Model file for the job. Use its own axes, mm. Face numbers are marked on the shaded views. Coordinates: 2 decimals unless noted, no trailing zeros. Order: outer loops, then holes, each group sorted by start corner. A loop starts at its lowest first (then second) coordinate and runs counter-clockwise, first axis right, second up. Notation, with made-up numbers: (16.5, 76.25) -> (53.5, 76.25) arc R22 ccw to (53.5, 96.25) -> close; hole circle Ø6 at (56.5, 85.25). An arc over 180 degrees is marked (long way). Write item = value, one per line. Start each with the question number.
Q1. Mould opens along X. For the marked faces 1, 2, 3 and 4 say: +X half, -X half, draft (parallel to the pull), parting line (faces both ways), or undercut.
Q2. Cut at A-A, the plane y = -2.25. List the corners of the cut face in (x, z), plus the area to 3 significant figures.
Q3. Cut at C-C, the plane x = -190.5. List the corners of the cut face in (y, z), plus the area to 4 significant figures.
Q4. Wall check: line 1 (X direction, y = 0.25, z = 3.25); line 2 (Z direction, x = -187, y = -2.5); line 3 (X direction, y = 0, z = 3.25). Give the ranges that are in metal, low to high. Write a range as from..to.
Q5. Flat gauge pin, fed straight in: pin 1 (1.5 mm diameter, centred on x = -181, z = 4.5, fed in from +Y). Where does the tip first touch, or does it go through?
Q6. Cut at D-D, the plane z = 4.5. Give the number of separate pieces and of enclosed holes in the cut face, plus the area to 3 significant figures.
Q7. Cut at B-B, the plane y = 8.25. List the corners of the cut face in (x, z).
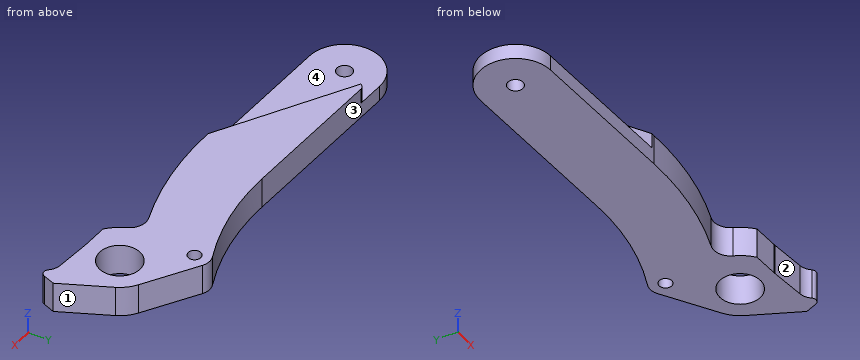
Autodesk Inventor part; units mm, degrees
ref_plane "YZ Plane" through (0, 0, 0) normal (1, 0, 0) x (0, 1, 0)
ref_plane "XZ Plane" through (0, 0, 0) normal (0, 1, 0) x (-1, 0, 0)
ref_plane "XY Plane" through (0, 0, 0) normal (0, 0, 1) x (1, 0, 0)
sketch "スケッチ1" plane through (0, 0, 0) normal (0, 0, 1) x (1, 0, 0)
  circle A0 centre (-145.5257, 0.5882) radius 1.5
  circle A1 centre (-139.5445, -10.0968) radius 1.5
  circle A2 centre (-105.5257, -16.4118) radius 30.1 construction
  line L0 (-170.915, -81.4118) -> (490.0044, -81.4118)
  circle A3 centre (-145.5257, 0.5882) radius 4.025
  circle A4 centre (-139.5445, -10.0968) radius 3
  circle A5 centre (-145.5257, 0.5882) radius 7.025
  line L1 (-146.2365, -6.4007) -> (-139.241, -7.1122)
  line L2 (-139.2044, 3.6529) -> (-134.6999, -5.6381)
  line L3 (-134.6999, -5.6381) -> (-136.7303, -11.1361)
  circle A6 centre (-105.5257, -16.4118) radius 31.1 construction
  line L4 (-145.1707, 7.6042) -> (-210.0877, 10.8882)
  line L5 (-145.8806, -6.4278) -> (-210.7976, -3.1438)
  circle A7 centre (-210.4427, 3.8722) radius 1.5
  circle A8 centre (-210.4427, 3.8722) radius 4.025
  circle A9 centre (-210.4427, 3.8722) radius 7.025
  circle A10 centre (-210.4427, 3.8722) radius 7.525
  line L6 (-206.5907, 10.3366) -> (-181.4786, -4.627)
  circle A11 centre (-199.4194, 13.3524) radius 1.25
  arc A12 (-199.5709, 10.3562) -> (-202.1936, 14.494) centre (-199.4194, 13.3524) ccw
  line L7 (-202.1936, 14.494) -> (-247.2482, 16.7732)
  arc A13 (-289.8377, 39.1951) -> (-247.2482, 16.7732) centre (-244.3571, 73.9244) ccw
  arc A14 (-289.8377, 39.1951) -> (-291.5649, 38.2266) centre (-290.6325, 38.5882) ccw
  arc A15 (-291.5649, 38.2266) -> (-251.8636, 4.9117) centre (-241.4172, 57.674) ccw
  line L8 (-251.8636, 4.9117) -> (-211.807, -3.019)
  line L9 (-209.3045, 11.3106) -> (-204.7936, 10.6204)
  arc A16 (-204.7936, 10.6204) -> (-205.5417, 8.9052) centre (-204.8441, 9.6217) ccw
  line L10 (-210.5022, 11.397) -> (-238.3358, 2.2334)
  point P0 (0, 0)
  point P1 (0, 0)
  point P2 (-146.0589, -6.4188)
  point P3 (-205.8121, 9.8726)
  dimension "d0" = 6
  dimension "d1" = 8.05
  dimension "d2" = 3
  dimension "d3" = 1
  dimension "d4" = 3
  dimension "d5" = 8.05
  dimension "d6" = 3
  dimension "d7" = 0.5
  dimension "d8" = 2.5
  dimension "d9" = 6
  dimension "d10" = 2
  dimension "d11" = 120
  dimension "d12" = 4
  dimension "d13" = 150
  dimension "d14" = 1
  dimension "d15" = 65
  dimension "d16" = 87.382
extrude "押し出し1" add sketch "スケッチ1" along normal blind 6 contours A4 L1 L5 A5 L2 L3 | L5 L6 A16 L4 A5 L1 | A5
extrude "押し出し2" add sketch "スケッチ1" along normal blind 3 contours L5 A10 A16 L6 | L5 A9 A16 A10 | A16 A10 L6 | L6 A10 L4 A16 | A9 | A10 A16 A9 L4 | A8
fillet "フィレット1" radius 1 1 edges at (-136.7303, -11.1361, 3)
sketch "スケッチ2" plane through (0, 0, 6) normal (0, 0, 1) x (1, 0, 0)
  line L0 (-210.7976, -3.1438) -> (-181.4786, -4.627)
  line L1 (-205.8121, 9.8726) -> (-181.4786, -4.627)
  arc A0 (-204.7936, 10.6204) -> (-205.8121, 9.8726) centre (-204.8441, 9.6217) ccw
  line L2 (-204.7936, 10.6204) -> (-210.0877, 10.8882)
  arc A1 (-210.0877, 10.8882) -> (-210.7976, -3.1438) centre (-210.4427, 3.8722) ccw
  circle A2 centre (-210.4427, 3.8722) radius 1.5
  arc A3 (-137.2374, -8.1793) -> (-135.5302, -7.8865) centre (-136.4683, -7.5401) ccw
  line L3 (-135.5302, -7.8865) -> (-134.6999, -5.6381)
  line L4 (-134.6999, -5.6381) -> (-139.2044, 3.6529)
  arc A4 (-139.2044, 3.6529) -> (-145.1707, 7.6042) centre (-145.5257, 0.5882) ccw
  line L5 (-145.1707, 7.6042) -> (-204.7936, 10.6204)
  arc A5 (-204.7936, 10.6204) -> (-205.8121, 9.8726) centre (-204.8441, 9.6217) ccw
  line L6 (-205.8121, 9.8726) -> (-181.4786, -4.627)
  line L7 (-181.4786, -4.627) -> (-146.0589, -6.4188)
  line L8 (-146.0589, -6.4188) -> (-146.2365, -6.4007)
  arc A6 (-146.2365, -6.4007) -> (-145.8806, -6.4278) centre (-145.5257, 0.5882) ccw
  line L9 (-145.8806, -6.4278) -> (-146.0589, -6.4188)
  line L10 (-146.0589, -6.4188) -> (-139.241, -7.1122)
  arc A7 (-137.2374, -8.1793) -> (-139.241, -7.1122) centre (-139.5445, -10.0968) ccw
  circle A8 centre (-145.5257, 0.5882) radius 4.025
  arc A9 (-204.7936, 10.6204) -> (-205.8121, 9.8726) centre (-204.8441, 9.6217) ccw
  line L11 (-204.6925, 12.6179) -> (-209.9867, 12.8857)
  arc A10 (-209.9867, 12.8857) -> (-210.8986, -5.1413) centre (-210.4427, 3.8722) ccw
  arc A11 (-182.0757, -6.5994) -> (-181.4786, -4.627) centre (-182.022, -5.539) ccw
  line L12 (-210.8986, -5.1413) -> (-182.0757, -6.5994)
  arc A12 (-204.7936, 10.6204) -> (-204.6925, 12.6179) centre (-204.743, 11.6191) ccw
  point P0 (0, 0)
  dimension "d22" = 2
sketch "スケッチ3" plane through (0, 0, 6) normal (0, 0, 1) x (1, 0, 0)
  arc A0 (-137.2374, -8.1793) -> (-135.5302, -7.8865) centre (-136.4683, -7.5401) ccw
  line L0 (-135.5302, -7.8865) -> (-134.6999, -5.6381)
  line L1 (-134.6999, -5.6381) -> (-139.2044, 3.6529)
  arc A1 (-139.2044, 3.6529) -> (-145.1707, 7.6042) centre (-145.5257, 0.5882) ccw
  line L2 (-145.1707, 7.6042) -> (-204.7936, 10.6204)
  arc A2 (-204.7936, 10.6204) -> (-205.8121, 9.8726) centre (-204.8441, 9.6217) ccw
  line L3 (-205.8121, 9.8726) -> (-181.4786, -4.627)
  line L4 (-181.4786, -4.627) -> (-146.0589, -6.4188)
  line L5 (-146.0589, -6.4188) -> (-146.2365, -6.4007)
  arc A3 (-146.2365, -6.4007) -> (-145.8806, -6.4278) centre (-145.5257, 0.5882) ccw
  line L6 (-145.8806, -6.4278) -> (-146.0589, -6.4188)
  line L7 (-146.0589, -6.4188) -> (-139.241, -7.1122)
  arc A4 (-137.2374, -8.1793) -> (-139.241, -7.1122) centre (-139.5445, -10.0968) ccw
  circle A5 centre (-145.5257, 0.5882) radius 4.025
  point P0 (0, 0)
extrude "押し出し3" add sketch "スケッチ3" against normal blind 6 contours L5 A3 L6
sketch "スケッチ4" plane through (0, 0, 6) normal (0, 0, 1) x (1, 0, 0)
  line L0 (-146.0589, -6.4188) -> (-139.241, -7.1122)
  arc A0 (-137.2374, -8.1793) -> (-139.241, -7.1122) centre (-139.5445, -10.0968) ccw
  arc A1 (-137.2374, -8.1793) -> (-135.5302, -7.8865) centre (-136.4683, -7.5401) ccw
  line L1 (-135.5302, -7.8865) -> (-134.6999, -5.6381)
  line L2 (-134.6999, -5.6381) -> (-139.2044, 3.6529)
  arc A2 (-139.2044, 3.6529) -> (-145.1707, 7.6042) centre (-145.5257, 0.5882) ccw
  line L3 (-145.1707, 7.6042) -> (-204.7936, 10.6204)
  arc A3 (-204.7936, 10.6204) -> (-205.8121, 9.8726) centre (-204.8441, 9.6217) ccw
  line L4 (-205.8121, 9.8726) -> (-181.4786, -4.627)
  line L5 (-181.4786, -4.627) -> (-146.0589, -6.4188)
  circle A4 centre (-145.5257, 0.5882) radius 4.025
  arc A5 (-153.4999, -3.002) -> (-157.5446, -1.2714) centre (-156.4634, -4.3363) ccw
  arc A6 (-180.854, -4.6586) -> (-157.5446, -1.2714) centre (-177.7808, 56.0903) ccw
  line L6 (-181.4786, -4.627) -> (-146.0589, -6.4188)
  circle A7 centre (-139.5445, -10.0968) radius 3
  arc A8 (-153.4999, -3.002) -> (-151.0823, -6.1647) centre (-145.5257, 0.5882) ccw
  line L7 (-145.1707, 7.6042) -> (-204.7936, 10.6204)
  arc A9 (-176.1768, 9.1728) -> (-154.4643, 13.0367) centre (-173.6978, 58.1782) ccw
  arc A10 (-151.6818, 12.8103) -> (-154.4643, 13.0367) centre (-153.2884, 10.2768) ccw
  line L8 (-151.6818, 12.8103) -> (-141.7636, 6.5209)
  circle A11 centre (-153.2884, 10.2768) radius 1.25
  circle A12 centre (-139.5445, -10.0968) radius 3.5
  point P0 (0, 0)
  point P1 (-176.1768, 9.1728)
  dimension "d25" = 3.25
  dimension "d26" = 95
  dimension "d27" = 3
  dimension "d28" = 2.5
  dimension "d29" = 0.5
extrude "押し出し4" cut sketch "スケッチ4" against normal blind 6 contours L5 A6 A5 A8
extrude "押し出し5" add sketch "スケッチ4" against normal blind 6 contours A2 L3 A9 A10 L8
sketch "スケッチ5" plane through (0, 0, 6) normal (0, 0, 1) x (1, 0, 0)
  circle A0 centre (-153.2884, 10.2768) radius 1.25
  circle A1 centre (-145.5257, 0.5882) radius 4.025
  arc A2 (-180.854, -4.6586) -> (-157.5446, -1.2714) centre (-177.7808, 56.0903) ccw
  arc A3 (-153.4999, -3.002) -> (-157.5446, -1.2714) centre (-156.4634, -4.3363) ccw
  arc A4 (-153.4999, -3.002) -> (-151.0823, -6.1647) centre (-145.5257, 0.5882) ccw
  line L0 (-151.0823, -6.1647) -> (-146.0589, -6.4188)
  line L1 (-146.0589, -6.4188) -> (-139.241, -7.1122)
  arc A5 (-137.2374, -8.1793) -> (-139.241, -7.1122) centre (-139.5445, -10.0968) ccw
  arc A6 (-137.2374, -8.1793) -> (-135.5302, -7.8865) centre (-136.4683, -7.5401) ccw
  line L2 (-135.5302, -7.8865) -> (-134.6999, -5.6381)
  line L3 (-134.6999, -5.6381) -> (-139.2044, 3.6529)
  arc A7 (-139.2044, 3.6529) -> (-141.7636, 6.5209) centre (-145.5257, 0.5882) ccw
  line L4 (-141.7636, 6.5209) -> (-151.6818, 12.8103)
  arc A8 (-151.6818, 12.8103) -> (-154.4643, 13.0367) centre (-153.2884, 10.2768) ccw
  arc A9 (-176.1768, 9.1728) -> (-154.4643, 13.0367) centre (-173.6978, 58.1782) ccw
  line L5 (-176.1768, 9.1728) -> (-204.7936, 10.6204)
  arc A10 (-204.7936, 10.6204) -> (-205.8121, 9.8726) centre (-204.8441, 9.6217) ccw
  line L6 (-205.8121, 9.8726) -> (-181.4786, -4.627)
  line L7 (-181.4786, -4.627) -> (-180.854, -4.6586)
  line L8 (-204.7936, 10.6204) -> (-210.0877, 10.8882)
  arc A11 (-210.0877, 10.8882) -> (-210.7976, -3.1438) centre (-210.4427, 3.8722) ccw
  line L9 (-210.7976, -3.1438) -> (-181.4786, -4.627)
  line L10 (-205.8121, 9.8726) -> (-181.4786, -4.627)
  arc A12 (-204.7936, 10.6204) -> (-205.8121, 9.8726) centre (-204.8441, 9.6217) ccw
  circle A13 centre (-210.4427, 3.8722) radius 1.5
  arc A14 (-204.7936, 10.6204) -> (-205.8121, 9.8726) centre (-204.8441, 9.6217) ccw
  arc A15 (-204.7936, 10.6204) -> (-204.6925, 12.6179) centre (-204.743, 11.6191) ccw
  line L11 (-204.6925, 12.6179) -> (-209.9867, 12.8857)
  arc A16 (-209.9867, 12.8857) -> (-210.8986, -5.1413) centre (-210.4427, 3.8722) ccw
  line L12 (-210.8986, -5.1413) -> (-182.0757, -6.5994)
  arc A17 (-182.0757, -6.5994) -> (-181.4786, -4.627) centre (-182.022, -5.539) ccw
  line L13 (-205.8121, 9.8726) -> (-181.4786, -4.627)
  point P0 (0, 0)
  dimension "d34" = 2
properties part number "後ろウイング根本" material "ポリカーボネート、クリア"
Here are the results:
q1.face_1 = +X half
q1.face_2 = -X half
q1.face_3 = undercut
q1.face_4 = draft
q2.outline = (-213.89, 0) -> (-160.57, 0) -> (-160.57, 6) -> (-185.47, 6) -> (-185.47, 3) -> (-213.89, 3) -> close; (-153.97, 0) -> (-148.38, 0) -> (-148.38, 6) -> (-153.97, 6) -> close; (-142.67, 0) -> (-136.34, 0) -> (-136.34, 6) -> (-142.67, 6) -> close
q2.area = 306 mm²
q3.outline = (-4.17, 0) -> (9.9, 0) -> (9.9, 6) -> (0.75, 6) -> (0.75, 3) -> (-4.17, 3) -> close
q3.area = 69.65 mm²
q4.line_1 = -189.66..-149.54, -141.51..-137.55
q4.line_2 = 0..3
q4.line_3 = -189.24..-149.51, -141.54..-137.43
q5.pin_1 = 9.45
q6.separate_pieces = 1
q6.enclosed_holes = 2
q6.area = 759 mm²
q7.outline = (-215.94, 0) -> (-144.49, 0) -> (-144.49, 6) -> (-203.09, 6) -> (-203.09, 3) -> (-215.94, 3) -> close
